Build history of the part. All positions in model axes, mm. Give positions to 0.01 mm unless a question says otherwise; leave off trailing zeros. Order: outer loops, then holes, each group sorted by start corner. A loop starts at its lowest first (then second) coordinate and runs counter-clockwise, first axis right, second up. Notation, with made-up numbers: (22, -14.75) - (46, -14.75) arc R15 ccw to (46, 4.25) - close; hole circle Ø4 at (31, 88.5). An arc over 180 degrees is marked (long way). Answer in a Markdown table with one row per item.
```python
from build123d import *

# Parameters (mm, degrees)
CROQUIS1_R              = 1
SALIENTE_EXTRUIR1_DEPTH = 3


with BuildPart() as part:
    # Croquis1 → Saliente-Extruir1 (new body)
    with BuildSketch(Plane.XY):
        Polygon((-34.480909091, -156.100114598), (-48.39, -156.100114598), (-48.39, -170.615828883), (-45.39, -170.615828883), (-45.39, -185.131543169), (-48.39, -185.131543169), (-48.39, -199.647257455), (-45.39, -199.647257455), (-45.39, -214.162971741), (-48.39, -214.162971741), (-48.39, -228.678686026), (-45.39, -228.678686026), (-45.39, -243.194400312), (-48.39, -243.194400312), (-48.39, -257.710114598), (-34.480909091, -257.710114598), (-34.480909091, -260.710114598), (-20.571818182, -260.710114598), (-20.571818182, -257.710114598), (-6.662727273, -257.710114598), (-6.662727273, -260.710114598), (7.246363636, -260.710114598), (7.246363636, -257.710114598), (21.155454545, -257.710114598), (21.155454545, -260.710114598), (35.064545455, -260.710114598), (35.064545455, -257.710114598), (48.973636364, -257.710114598), (48.973636364, -260.710114598), (62.882727273, -260.710114598), (62.882727273, -257.710114598), (76.791818182, -257.710114598), (76.791818182, -260.710114598), (90.700909091, -260.710114598), (90.700909091, -257.710114598), (104.61, -257.710114598), (104.61, -243.087661526), (101.61, -243.087661526), (101.61, -228.678686026), (104.61, -228.678686026), (104.61, -214.162971741), (101.61, -214.162971741), (101.61, -199.647257455), (104.61, -199.647257455), (104.61, -185.131543169), (101.61, -185.131543169), (101.61, -170.615828883), (104.61, -170.615828883), (104.61, -156.100114598), (90.700909091, -156.100114598), (90.700909091, -153.100114598), (76.791818182, -153.100114598), (76.791818182, -156.100114598), (62.882727273, -156.100114598), (62.882727273, -153.100114598), (48.973636364, -153.100114598), (48.973636364, -156.100114598), (35.440889541, -156.100114598), (35.440889541, -153.100114598), (21.155454545, -153.100114598), (21.155454545, -156.100114598), (7.246363636, -156.100114598), (7.246363636, -153.100114598), (-6.662727273, -153.100114598), (-6.662727273, -156.100114598), (-20.571818182, -156.100114598), (-20.571818182, -153.100114598), (-34.480909091, -153.100114598), align=None)
        with Locations((99.61, -168.670114598)):
            Circle(CROQUIS1_R, mode=Mode.SUBTRACT)
        with Locations((99.61, -204.670114598)):
            Circle(CROQUIS1_R, mode=Mode.SUBTRACT)
        with Locations((43.61, -168.670114598)):
            Circle(CROQUIS1_R, mode=Mode.SUBTRACT)
        with Locations((43.61, -204.670114598)):
            Circle(CROQUIS1_R, mode=Mode.SUBTRACT)
    extrude(amount=SALIENTE_EXTRUIR1_DEPTH)


solid = part.part
```
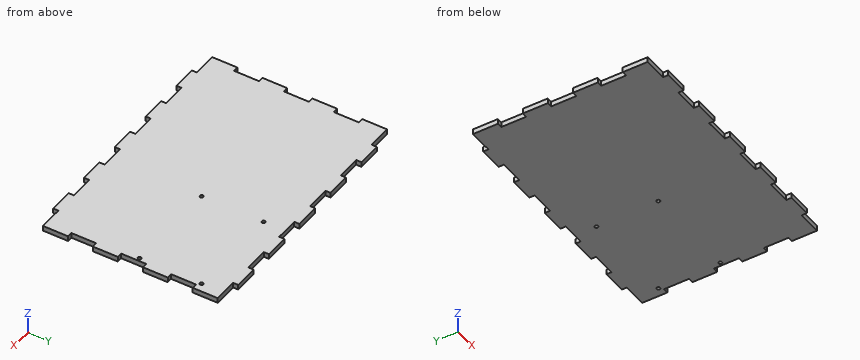
1. Cut at C-C on x = 12. Write the cut outline in (y, z).
Check result:
| item | result |
|---|---|
| outline | (-257.71, 0) - (-156.1, 0) - (-156.1, 3) - (-257.71, 3) - close |
2. Cut at A-A on z = 2.55. Count the separate pieces of the cut face and the enclosed holes in it, and give its area (3 significant figures).
Check result:
| item | result |
|---|---|
| separate pieces | 1 |
| enclosed holes | 4 |
| area | 15,700 mm² |
3. Drop flat-ended pins along their axis: P1, Ø1.5, axis at y = -259.5, z = 1.5, coming from the +X side; P2, Ø1.5, axis at y = -258.5, z = 2, coming from the -X side; P3, Ø0.9, axis at x = -47, z = 1, coming from the -Y side. Give the stop position or say it passes through.
Check result:
| item | result |
|---|---|
| P1 | stops at x = 90.7 |
| P2 | stops at x = -34.48 |
| P3 | stops at y = -257.71 |
4. Probe line 1 (Y direction, x = 43.61, z = 1.25); line 2 (Y direction, x = -35, z = 0.5); line 3 (X direction, y = -202.5, z = 0.25). List the from-to ranges inside material, lowest first.
Check result:
| item | result |
|---|---|
| line 1 | y = -257.71 to -205.67, -203.67 to -169.67, -167.67 to -156.1 |
| line 2 | y = -257.71 to -156.1 |
| line 3 | x = -45.39 to 101.61 |
5. Cut at B-B on y = -182.5. Write the cut outline in (x, z).
Check result:
| item | result |
|---|---|
| outline | (-45.39, 0) - (101.61, 0) - (101.61, 3) - (-45.39, 3) - close |
